Read the model definition and answer for the solid it produces. Units are mm, in the model's axes. A direction names the side the tool comes from. Give positions to 0.01 mm unless a question says otherwise; leave off trailing zeros. Loops run counter-clockwise (first coordinate to the right, second up) from the corner with the lowest first, then second, coordinate; pieces in that order, holes last.
(1) Determine the mould class of faces 3 (the face through (0, 32, 1)), 4 (the face through (4.056, 53.083, -3.351)), 5 (the face through (35, 8, 1)) for opening direction Y: pulls with the +Y half, pulls with the -Y half, needs draft (parallel to the pull), parting line crosses it, or undercut.
(2) Find section C-C, the plane x = 46. Write down the section's boundary in (y, z).
(3) Find section A-A, the plane z = 0. Write down the section's boundary in (x, y), then the cut area to 3 significant figures.
(4) Find section B-B, the plane y = 45. Write down the section's boundary in (x, z).
(5) Which of the six approach directions +Z, -Z, +X, -X, +Y, -Y give full straight-line access (tool end or side, diameter ignored) to faces 1 (the face through (46.9, 4.06, -8.54)), 2 (the face through (8, 55, 1))?
(6) Find section D-D, the plane y = 57. Write down the section's boundary in (x, z).
(7) Each of these flat-tipped pins is pushed along its axis until it touches: P1, Ø10, axis at y = 39, z = -29.5, coming from the +X side; P2, Ø6, axis at x = 39, z = -28.5, coming from the +Y side. Where does it stop, or does it pass through?
(8) Straight lines are drawn through the part: probe 1 along Y at (x, z) = (24, -2); probe 2 along Z at (x, y) = (5.25, 45). For each, find the intervals that lie inside material, in ascending order.
```python
from build123d import *

# Parameters (mm, degrees)
AUFSATZ_AUFTRAGEN_MAIN_BODY_DEPTH = 40
SKIZZE3_R                         = 8.75
BOHRUNG_HORIZONTAL_DEPTH          = 115.821600755
SKIZZE4_R                         = 8.75
BOHRUNG_VERTIKAL_DEPTH            = 115.821600755
LINEAR_AUSTRAGEN_DEPTH            = 115.821600755
VERRUNDUNG_R                      = 5


with BuildPart() as part:
    # Skizze1 → Aufsatz Auftragen Main Body (new, symmetric)
    with BuildSketch(Plane.XY):
        with BuildLine():
            Line((0, 0), (80, 0))
            Line((80, 0), (80, 8))
            Line((80, 8), (18, 8))
            ThreePointArc((18, 8), (10.928932188, 10.928932188), (8, 18))
            Line((8, 18), (8, 80))
            Line((8, 80), (0, 80))
            Line((0, 80), (0, 0))
        make_face()
    extrude(amount=AUFSATZ_AUFTRAGEN_MAIN_BODY_DEPTH, both=True)

    # Skizze3 → Bohrung Horizontal (cut, through all)
    with BuildSketch(Plane(origin=(0, 8, 0), x_dir=(1, 0, 0), z_dir=(0, 1, 0))):
        with Locations(Location((45, 0, 0), (0, 0, 180))):
            Circle(SKIZZE3_R)
    extrude(amount=-BOHRUNG_HORIZONTAL_DEPTH, mode=Mode.SUBTRACT)

    # Skizze4 → Bohrung Vertikal (cut, through all)
    with BuildSketch(Plane(origin=(8, 0, 0), x_dir=(0, 0, -1), z_dir=(1, 0, 0))):
        with Locations(Location((0, 45, 0), (0, 0, 90))):
            Circle(SKIZZE4_R)
    extrude(amount=-BOHRUNG_VERTIKAL_DEPTH, mode=Mode.SUBTRACT)

    # Skizze5 → Linear Austragen (cut, through all)
    with BuildSketch(Plane(origin=(0, 8, 0), x_dir=(1, 0, 0), z_dir=(0, 1, 0))):
        with BuildLine():
            Line((24, -40), (55.971921298, -12.985258682))
            ThreePointArc((55.971921298, -12.985258682), (62, 0), (55.971921298, 12.985258682))
            Line((55.971921298, 12.985258682), (24, 40))
            Line((24, 40), (80, 40))
            Line((80, 40), (80, -40))
            Line((80, -40), (24, -40))
        make_face()
    extrude(amount=-LINEAR_AUSTRAGEN_DEPTH, mode=Mode.SUBTRACT)

    # Verrundung
    verrundung_edges = [part.edges().sort_by_distance(p)[0] for p in [
        (24, 4, 40),
        (24, 4, -40),
    ]]
    fillet(verrundung_edges, radius=VERRUNDUNG_R)


solid = part.part
```
Entries:
1. face 3: needs draft
1. face 4: undercut
1. face 5: pulls with the +Y half
2. outline: (0, -21.41) - (8, -21.41) - (8, -8.69) - (0, -8.69) - close; (0, 8.69) - (8, 8.69) - (8, 21.41) - (0, 21.41) - close
3. outline: (0, 0) - (36.25, 0) - (36.25, 8) - (18, 8) arc R10 cw to (8, 18) - (8, 36.25) - (0, 36.25) - close; (0, 53.75) - (8, 53.75) - (8, 80) - (0, 80) - close; (53.75, 0) - (62, 0) - (62, 8) - (53.75, 8) - close
3. area: 813 mm2
4. outline: (0, -40) - (8, -40) - (8, -8.75) - (0, -8.75) - close; (0, 8.75) - (8, 8.75) - (8, 40) - (0, 40) - close
5. face 1: +Y, -Y
5. face 2: +Z, -Z, +X, +Y
6. outline: (0, -40) - (8, -40) - (8, 40) - (0, 40) - close
7. P1: stops at x = 8
7. P2: stops at y = 8
8. probe 1: y = 0 to 8
8. probe 2: z = -40 to -8.75, 8.75 to 40
